from build123d import *

# Parameters (mm, degrees)
SKETCH1_R           = 16.5
BOSS_EXTRUDE1_DEPTH = 3
SKETCH2_R           = 4.5
BOSS_EXTRUDE2_DEPTH = 2
CUT_EXTRUDE1_DEPTH  = 24.526580712
CIRPATTERN1_COUNT   = 4
SKETCH4_R           = 16
BOSS_EXTRUDE3_DEPTH = 2.5
CUT_EXTRUDE2_DEPTH  = 24.973944189
CIRPATTERN2_COUNT   = 2
CUT_EXTRUDE3_DEPTH  = 24.973944189
CIRPATTERN3_COUNT   = 2
SKETCH8_R           = 1.45
CUT_EXTRUDE4_DEPTH  = 0.5
SKETCH9_W           = 0.5
SKETCH9_H           = 2.9
EXTRUDE_THIN1_DEPTH = 0.5
SKETCH10_W          = 2.9
SKETCH10_H          = 0.5
EXTRUDE_THIN2_DEPTH = 0.5
SKETCH11_W          = 3
SKETCH11_H          = 0.6
CUT_EXTRUDE5_DEPTH  = 24.973944189
CIRPATTERN4_COUNT   = 2
FILLET1_R           = 0.1
FILLET2_R           = 0.5
SKETCH_1_R          = 1.5
EXTRUDE_1_DEPTH     = 2


with BuildPart() as part:
    # Sketch1 → Boss-Extrude1 (new body)
    with BuildSketch(Plane.XY):
        Circle(SKETCH1_R)
    extrude(amount=-BOSS_EXTRUDE1_DEPTH)

    # Sketch2 → Boss-Extrude2 (add)
    with BuildSketch(Plane(origin=(0, 0, -3), x_dir=(-1, 0, 0), z_dir=(0, 0, -1))):
        Circle(SKETCH2_R)
    extrude(amount=BOSS_EXTRUDE2_DEPTH)

    # Sketch3 → Cut-Extrude1 (cut, through all)
    with BuildSketch(Plane(origin=(0, 0, -3), x_dir=(-1, 0, 0), z_dir=(0, 0, -1))):
        Polygon((10.253048327, 13.081475452), (8.131727984, 10.960155108), (10.960155108, 8.131727984), (13.081475452, 10.253048327), align=None)
    cut_extrude1 = extrude(amount=-CUT_EXTRUDE1_DEPTH, mode=Mode.SUBTRACT)

    # CirPattern1: Cut-Extrude1 ×4 about axis
    cirpattern1_axis = Axis((0, 0, 0), (0, 0, 1))
    for i in range(1, CIRPATTERN1_COUNT):
        add(cut_extrude1.rotate(cirpattern1_axis, i * 360 / CIRPATTERN1_COUNT), mode=Mode.SUBTRACT)

    # Sketch4 → Boss-Extrude3 (add)
    with BuildSketch(Plane.XY):
        with Locations(Location((0, 0, 0), (0, 0, 217.819244219))):
            Circle(SKETCH4_R)
    extrude(amount=BOSS_EXTRUDE3_DEPTH)

    # Sketch6 → Cut-Extrude2 (cut, through all)
    with BuildSketch(Plane(origin=(0, 0, -3), x_dir=(-1, 0, 0), z_dir=(0, 0, -1))):
        with BuildLine():
            Line((-4.67653718, 2.7), (-3.810511777, 2.2))
            ThreePointArc((-3.810511777, 2.2), (-4.4, 0), (-3.810511777, -2.2))
            Line((-3.810511777, -2.2), (-4.67653718, -2.7))
            ThreePointArc((-4.67653718, -2.7), (-5.4, 0), (-4.67653718, 2.7))
        make_face()
    cut_extrude2 = extrude(amount=-CUT_EXTRUDE2_DEPTH, mode=Mode.SUBTRACT)

    # CirPattern2: Cut-Extrude2 ×2 about axis
    cirpattern2_axis = Axis((0, 0, 0), (0, 0, 1))
    for i in range(1, CIRPATTERN2_COUNT):
        add(cut_extrude2.rotate(cirpattern2_axis, i * 360 / CIRPATTERN2_COUNT), mode=Mode.SUBTRACT)

    # Sketch7 → Cut-Extrude3 (cut, through all)
    with BuildSketch(Plane(origin=(0, 0, -3), x_dir=(-1, 0, 0), z_dir=(0, 0, -1))):
        with BuildLine():
            ThreePointArc((2.223130932, 6.108002035), (0, 6.5), (-2.223130932, 6.108002035))
            ThreePointArc((-2.223130932, 6.108002035), (-2.67138529, 5.146717462), (-1.710100717, 4.698463104))
            ThreePointArc((-1.710100717, 4.698463104), (0, 5), (1.710100717, 4.698463104))
            ThreePointArc((1.710100717, 4.698463104), (2.67138529, 5.146717462), (2.223130932, 6.108002035))
        make_face()
    cut_extrude3 = extrude(amount=-CUT_EXTRUDE3_DEPTH, mode=Mode.SUBTRACT)

    # CirPattern3: Cut-Extrude3 ×2 about axis
    cirpattern3_axis = Axis((0, 0, 0), (0, 0, 1))
    for i in range(1, CIRPATTERN3_COUNT):
        add(cut_extrude3.rotate(cirpattern3_axis, i * 360 / CIRPATTERN3_COUNT), mode=Mode.SUBTRACT)

    # Sketch8 → Cut-Extrude4 (cut)
    with BuildSketch(Plane(origin=(0, 0, -3), x_dir=(-1, 0, 0), z_dir=(0, 0, -1))):
        with Locations((-7.071067812, 7.071067812)):
            Circle(SKETCH8_R)
        Polygon((8.485281374, -3.535533906), (3.535533906, -8.485281374), (5.656854249, -10.606601718), (10.606601718, -5.656854249), align=None)
    extrude(amount=-CUT_EXTRUDE4_DEPTH, mode=Mode.SUBTRACT)

    # Sketch9 → Extrude-Thin1 (add)
    with BuildSketch(Plane(origin=(0, 0, -2.5), x_dir=(-1, 0, 0), z_dir=(0, 0, -1))):
        with Locations((-7.071067812, 7.071067812)):
            Rectangle(SKETCH9_W, SKETCH9_H)
    extrude(amount=EXTRUDE_THIN1_DEPTH)

    # Sketch10 → Extrude-Thin2 (add)
    with BuildSketch(Plane(origin=(0, 0, -2.5), x_dir=(-1, 0, 0), z_dir=(0, 0, -1))):
        with Locations((-7.071067812, 7.071067812)):
            Rectangle(SKETCH10_W, SKETCH10_H)
    extrude(amount=EXTRUDE_THIN2_DEPTH)

    # Sketch11 → Cut-Extrude5 (cut, through all)
    with BuildSketch(Plane(origin=(0, 0, -3), x_dir=(-1, 0, 0), z_dir=(0, 0, -1))):
        with Locations((0, 12.8)):
            Rectangle(SKETCH11_W, SKETCH11_H)
    cut_extrude5 = extrude(amount=-CUT_EXTRUDE5_DEPTH, mode=Mode.SUBTRACT)

    # CirPattern4: Cut-Extrude5 ×2 about axis
    cirpattern4_axis = Axis((0, 0, 0), (0, 0, 1))
    for i in range(1, CIRPATTERN4_COUNT):
        add(cut_extrude5.rotate(cirpattern4_axis, i * 360 / CIRPATTERN4_COUNT), mode=Mode.SUBTRACT)

    # Fillet1
    # the kernel refuses this fillet: 0.1 mm, written as the material it adds along each edge
    with BuildSketch(Plane(origin=(0, 0, -3), x_dir=(0.86602540378442, -0.5000000000000324, 0), z_dir=(0.5000000000000324, 0.86602540378442, 0))) as fillet1_piece_1:
        with BuildLine():
            CenterArc((4.5 + FILLET1_R, FILLET1_R), FILLET1_R, 180, 90)
            Line((4.5, FILLET1_R), (4.5, 0))
            Line((4.5, 0), (4.5 + FILLET1_R, 0))
        make_face()
    revolve(axis=Axis((0, 0, -3), (0, 0, -1)), revolution_arc=120)
    with BuildSketch(Plane(origin=(0, 0, -3), x_dir=(-0.8660254037844196, 0.500000000000033, 0), z_dir=(-0.500000000000033, -0.8660254037844196, 0))) as fillet1_piece_2:
        with BuildLine():
            CenterArc((4.5 + FILLET1_R, FILLET1_R), FILLET1_R, 180, 90)
            Line((4.5, FILLET1_R), (4.5, 0))
            Line((4.5, 0), (4.5 + FILLET1_R, 0))
        make_face()
    revolve(axis=Axis((0, 0, -3), (0, 0, -1)), revolution_arc=120)
    # the kernel refuses this fillet: 0.1 mm, written as the material it takes off along each edge
    with BuildSketch(Plane(origin=(0, 0, -5), x_dir=(-1, 0, 0), z_dir=(0, -1, 0))) as fillet1_2_piece_1:
        with BuildLine():
            CenterArc((4.5 - FILLET1_R, -FILLET1_R), FILLET1_R, 0, 90)
            Line((4.5 - FILLET1_R, 0), (4.5, 0))
            Line((4.5, 0), (4.5, -FILLET1_R))
        make_face()
    revolve(axis=Axis((0, 0, -5), (0, 0, -1)), mode=Mode.SUBTRACT)

    # Fillet2
    fillet2_edges = [part.edges().sort_by_distance(p)[0] for p in [
        (-16.5, 0, -3),
        (0, -16.5, -3),
        (16.5, 0, -3),
        (0, 16.5, -3),
    ]]
    fillet(fillet2_edges, radius=FILLET2_R)

    # Эскиз1 → Бобышка-Вытянуть1 (add)
    with BuildSketch(Plane(origin=(0, 0, -5), x_dir=(-1, 0, 0), z_dir=(0, 0, -1))):
        Circle(SKETCH_1_R)
    extrude(amount=EXTRUDE_1_DEPTH)


solid = part.part
CAD build for the part. Positions are in the model's coordinates, mm. A direction names the side the tool comes from. Give positions to 0.01 mm unless a question says otherwise; leave off trailing zeros. Loops run counter-clockwise (first coordinate to the right, second up) from the corner with the lowest first, then second, coordinate; pieces in that order, holes last. Notation, with made-up numbers: M 81,-13 L 116,-13 A15 ccw 116,-2 Z; hole C 36,20.25 d2. An arc over 180 degrees is marked long. Answer in a Markdown table with one row per item. Add a question column.
Item 1: Band-saw the part on B-B on x = 0. Give the number of separate pieces and of enclosed holes in the cut face, then the cut area to 3 significant figures.
Item 2: Band-saw the part on C-C on z = -3.5. Give the cut face in (x, y), then the cut area to 3 significant figures.
Item 3: Band-saw the part on A-A on y = 0. Give the cut face in (x, z).
Item 4: Drop flat-ended pins along their axis: P1, Ø1.3, axis at x = 6.5, y = 6.5, coming from the -Z side; P2, Ø0.5, axis at y = -13, z = 1, coming from the +X side; P3, Ø5, axis at x = -11.5, z = -3, coming from the -Y side. Give the stop position or say it passes through.
Item 5: Probe probe 1 along Y at (x, z) = (9, -1); probe 2 along Y at (x, z) = (2, 1.5); probe 3 along Y at (x, z) = (-8.5, -2.75). List the from-to ranges inside material, lowest first.
Item 6: Tool access for faces 1 (the face through (1.5, 0.07, -5.99)), 2 (the face through (0, 16.2, 0)), 3 (the face through (5.4, 0, -0.3)): list every direction of +Z, -Z, +X, -X, +Y, -Y with a clear straight run to the whole face (end or side of a thin tool).
Item 7: Mould opens along X. For faces 4 (the face through (3, 4, -3)), 5 (the face through (-9.135, -11.964, -1.521)), 6 (the face through (-9.526, 9.566, -1.521)) say: +X half, -X half, draft (parallel to the pull), parting line (faces both ways), or undercut.
Reply:
| question | item | result |
|---|---|---|
| 1 | separate pieces | 5 |
| 1 | enclosed holes | 0 |
| 1 | area | 180 mm^2 |
| 2 | outline | C 0,0 d9 |
| 2 | area | 63.6 mm^2 |
| 3 | outline | M -16.5,-2.5 A0.5 ccw -16,-3 L -5.4,-3 L -5.4,2.5 L -16,2.5 L -16,0 L -16.5,0 Z; M -4.5,-4.9 A0.1 ccw -4.4,-5 L -1.5,-5 L -1.5,-7 L 1.5,-7 L 1.5,-5 L 4.4,-5 A0.1 ccw 4.5,-4.9 L 4.5,-3 L 4.4,-3 L 4.4,2.5 L -4.4,2.5 L -4.4,-3 L -4.5,-3 Z; M 5.4,-3 L 16,-3 A0.5 ccw 16.5,-2.5 L 16.5,0 L 16,0 L 16,2.5 L 5.4,2.5 Z |
| 4 | P1 | stops at z = -3 |
| 4 | P2 | stops at x = 9.67 |
| 4 | P3 | stops at y = -13.8 |
| 5 | probe 1 | y = -13.83 to -11.83, -10.09 to 10.09, 11.83 to 13.83 |
| 5 | probe 2 | y = -15.87 to -6.18, -4.65 to 4.65, 6.18 to 15.87 |
| 5 | probe 3 | y = -14.06 to -11.33, -10.59 to -7.76, -3.55 to 10.59, 11.33 to 14.06 |
| 6 | face 1 | -Z |
| 6 | face 2 | +Z, +Y |
| 6 | face 3 | +Z, -Z |
| 7 | face 4 | draft |
| 7 | face 5 | -X half |
| 7 | face 6 | undercut |
